Verification items for the finished model (mm, model axes). Coordinates: 2 decimals unless noted, no trailing zeros. Write each loop counter-clockwise with the first axis right and the second up, starting at its lowest first coordinate (ties: lowest second). Pieces come first, ordered by that corner, then holes. Notation, with made-up numbers: (-24, 63.25) -> (18, 63.25) arc R35 cw to (18, 97.25) -> close; hole circle Ø5 at (37.25, 5). An arc over 180 degrees is marked (long way). Use a Markdown table: item, result. Add a question column.
from build123d import *

# Parameters (mm, degrees)
BASE_FLANGE1_DEPTH = 6


# Sheet-metal steps are written as plain solids
with BuildPart() as part:
    # Sketch1 → Base-Flange1 (new body)
    with BuildSketch(Plane(origin=(0, 0, 0), x_dir=(0, 0, -1), z_dir=(1, 0, 0))):
        with BuildLine():
            Line((-31.859064644, 3), (-260, 3))
            Line((-260, 3), (-260, 18))
            Line((-260, 18), (-30, 80))
            Line((-30, 80), (30, 80))
            Line((30, 80), (280, 18))
            Line((280, 18), (280, 3))
            Line((280, 3), (31.859064644, 3))
            ThreePointArc((31.859064644, 3), (0, 32), (-31.859064644, 3))
        make_face()
    extrude(amount=-BASE_FLANGE1_DEPTH)


solid = part.part
1) Gauge pin test, flat end, axial feed: pin 1 (4 mm diameter, centred on y = 63.5, z = -108.5, fed in from -X). Record the tip position at first contact, or that the pin passes through.
2) Release check for a two-part mould opening along Z. For faces 1 (the face through (-2.958, 31.993, -0.662)), 2 (the face through (0, 33, -14)), 3 (the face through (-2.958, 49.434, -153.25)) record: released by +Z, released by -Z, zero draft, split by the parting line, or undercut.
3) Cross-section at C-C on z = -196. Record the boundary of the cut face in (x, y).
4) Thickness scan on L1, parallel to Z at x = -1.6, y = 16; L2, parallel to Y at x = -5.4, z = 0.5; L3, parallel to Y at x = -1.9, z = -18. Record the ranges inside material, lowest first.
5) Cross-section at B-B on y = 62. Record the boundary of the cut face in (x, z), then the cut area to 3 significant figures.
6) Cross-section at A-A on x = -4.15. Record the boundary of the cut face in (y, z), then the cut area to 3 significant figures.
Returned:
| question | item | result |
|---|---|---|
| 1 | pin 1 | passes through |
| 2 | face 1 | undercut |
| 2 | face 2 | zero draft |
| 2 | face 3 | released by -Z |
| 3 | outline | (-6, 3) -> (0, 3) -> (0, 38.83) -> (-6, 38.83) -> close |
| 4 | L1 | z = -280 to -27.71, 27.71 to 260 |
| 4 | L2 | y = 32 to 80 |
| 4 | L3 | y = 26.46 to 80 |
| 5 | outline | (-6, -102.58) -> (0, -102.58) -> (0, 96.77) -> (-6, 96.77) -> close |
| 5 | area | 1,200 mm² |
| 6 | outline | (3, -280) -> (18, -280) -> (80, -30) -> (80, 30) -> (18, 260) -> (3, 260) -> (3, 31.86) arc R32 cw to (3, -31.86) -> close |
| 6 | area | 25,300 mm² |
